CAD build for the part. Positions are in the model's coordinates, mm. Face numbers are marked on the shaded views. A direction names the side the tool comes from. Round coordinates to 2 decimals unless told otherwise and drop trailing zeros. Write each loop counter-clockwise with the first axis right and the second up, starting at its lowest first coordinate (ties: lowest second). Pieces come first, ordered by that corner, then holes. Notation, with made-up numbers: (-18, 83.5) - (26, 83.5) arc R25 cw to (26, 106.5) - close; hole circle Ø3 at (34, -25). An arc over 180 degrees is marked (long way). Answer in a Markdown table with one row per item.
```python
from build123d import *

# Parameters (mm, degrees)
SKETCH1_W               = 402.68
SKETCH1_H               = 30
BOSS_EXTRUDE1_DEPTH     = 2.03
SKETCH2_W               = 402.68
SKETCH2_H               = 30
BOSS_EXTRUDE2_DEPTH     = 2.03
CONVERT_SOLID1_START    = -201.34
CONVERT_SOLID1_DEPTH    = 402.68
CONVERT_SOLID1_2_DEPTH  = 402.68
CUT_EXTRUDE1_START      = -201.34
CUT_EXTRUDE1_DEPTH      = 75
CUT_EXTRUDE1_START_2    = 126.34
CUT_EXTRUDE1_2_DEPTH    = 75
CUT_EXTRUDE2_DEPTH      = 239.296116766
CUT_EXTRUDE2_DEPTH_BACK = 239.296116766
SKETCH8_R               = 3.1
CUT_EXTRUDE3_DEPTH      = 239.27017557
CUT_EXTRUDE3_DEPTH_BACK = 239.27017557
SKETCH10_R              = 3.1


# Read off the part's stored shape, not the designer's step: Convert-Solid1, Cut-Extrude1
with BuildPart() as part:
    # Sketch1 → Boss-Extrude1 (new body)
    with BuildSketch(Plane(origin=(0, 0, 0), x_dir=(1, 0, 0), z_dir=(0, 1, 0))):
        Rectangle(SKETCH1_W, SKETCH1_H)
    extrude(amount=BOSS_EXTRUDE1_DEPTH)


with BuildPart() as body_2:
    # Sketch2 → Boss-Extrude2 (new body)
    with BuildSketch(Plane(origin=(0, 0, 0), x_dir=(1, 0, 0), z_dir=(0, 1, 0))):
        with Locations((0, 112.4)):
            Rectangle(SKETCH2_W, SKETCH2_H)
    extrude(amount=-BOSS_EXTRUDE2_DEPTH)


    add(part.part)  # loft1 joins it to this body
    # loft from a face of the part (loft1)
    loft([body_2.faces().sort_by_distance((0, -1.015, -97.4))[0], body_2.faces().sort_by_distance((0, 1.015, -15))[0]])

    # Convert-Solid1 outline → Convert-Solid1 (cut)
    with BuildSketch(Plane.YZ.offset(CONVERT_SOLID1_START)):
        with BuildLine():
            ThreePointArc((2.03, -14.851837405), (2.029087712, -14.999988764), (2.026350985, -15.148117654))
            Line((2.026350985, -15.148117654), (2.03, -15))
            Line((2.03, -15), (2.03, -14.851837405))
        make_face()
        with BuildLine():
            ThreePointArc((-2.03, -97.523160927), (-2.029683266, -97.435865309), (-2.02873308, -97.348574287))
            Line((-2.02873308, -97.348574287), (-2.03, -97.4))
            Line((-2.03, -97.4), (-2.03, -97.523160927))
        make_face()
    extrude(amount=CONVERT_SOLID1_DEPTH, mode=Mode.SUBTRACT)

    # Convert-Solid1 2 outline → Convert-Solid1 2 (add)
    with BuildSketch(Plane.YZ.offset(CONVERT_SOLID1_START)):
        with BuildLine():
            Line((0, -97.4), (0, -97.523160927))
            ThreePointArc((0, -97.523160927), (0.000758344, -97.40000934), (0.003033263, -97.276876431))
            Line((0.003033263, -97.276876431), (0, -97.4))
        make_face()
        with BuildLine():
            ThreePointArc((0, -14.851837405), (-0.000758344, -14.974988992), (-0.003033263, -15.098121901))
            Line((-0.003033263, -15.098121901), (-2.026350985, -97.226880678))
            ThreePointArc((-2.026350985, -97.226880678), (-2.027695942, -97.28772447), (-2.02873308, -97.348574287))
            Line((-2.02873308, -97.348574287), (0, -15))
            Line((0, -15), (0, -14.851837405))
        make_face()
    extrude(amount=CONVERT_SOLID1_2_DEPTH)

    # Cut-Extrude1 outline → Cut-Extrude1 (cut)
    with BuildSketch(Plane.YZ.offset(CUT_EXTRUDE1_START)):
        with BuildLine():
            Line((-0.003033263, -15.098121901), (-1.508642262, -76.212497042))
            Line((-1.508642262, -76.212497042), (0.520741986, -76.262492795))
            Line((0.520741986, -76.262492795), (2.026350985, -15.148117654))
            ThreePointArc((2.026350985, -15.148117654), (2.029087712, -14.999988764), (2.03, -14.851837405))
            Line((2.03, -14.851837405), (2.03, -6.212497042))
            Line((2.03, -6.212497042), (0, -6.212497042))
            Line((0, -6.212497042), (0, -14.851837405))
            ThreePointArc((0, -14.851837405), (-0.000758344, -14.974988992), (-0.003033263, -15.098121901))
        make_face()
    extrude(amount=CUT_EXTRUDE1_DEPTH, mode=Mode.SUBTRACT)

    # Cut-Extrude1 2 outline → Cut-Extrude1 2 (cut)
    with BuildSketch(Plane.YZ.offset(CUT_EXTRUDE1_START_2)):
        with BuildLine():
            Line((-0.003033263, -15.098121901), (-1.508642262, -76.212497042))
            Line((-1.508642262, -76.212497042), (0.520741986, -76.262492795))
            Line((0.520741986, -76.262492795), (2.026350985, -15.148117654))
            ThreePointArc((2.026350985, -15.148117654), (2.029087712, -14.999988764), (2.03, -14.851837405))
            Line((2.03, -14.851837405), (2.03, -6.212497042))
            Line((2.03, -6.212497042), (0, -6.212497042))
            Line((0, -6.212497042), (0, -14.851837405))
            ThreePointArc((0, -14.851837405), (-0.000758344, -14.974988992), (-0.003033263, -15.098121901))
        make_face()
    extrude(amount=CUT_EXTRUDE1_2_DEPTH, mode=Mode.SUBTRACT)

    # Sketch8 → Cut-Extrude2 (cut, two sides: drawn at the far end of the back side and taken through both)
    with BuildSketch(Plane.XZ.offset(2.03).offset(-CUT_EXTRUDE2_DEPTH_BACK)):
        with Locations(Location((95.117, -114.9, 0), (0, 0, 270))):
            Circle(SKETCH8_R)
        with Locations(Location((-95.117, -114.9, 0), (0, 0, 270))):
            Circle(SKETCH8_R)
    extrude(amount=CUT_EXTRUDE2_DEPTH + CUT_EXTRUDE2_DEPTH_BACK, mode=Mode.SUBTRACT)

    # Sketch10 → Cut-Extrude3 (cut, two sides: drawn at the far end of the back side and taken through both)
    with BuildSketch(Plane.XZ.offset(-CUT_EXTRUDE3_DEPTH_BACK)):
        with Locations(Location((95.116996944, 2.5, 0), (0, 0, 270))):
            Circle(SKETCH10_R)
        with Locations(Location((-95.117, 2.5, 0), (0, 0, 270))):
            Circle(SKETCH10_R)
    extrude(amount=CUT_EXTRUDE3_DEPTH + CUT_EXTRUDE3_DEPTH_BACK, mode=Mode.SUBTRACT)


solid = body_2.part
```
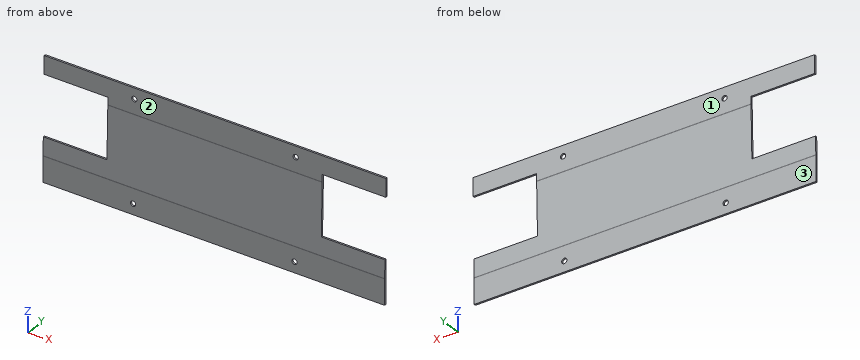
Q1. Saw through at D-D on z = -60. List the corners of the cut face in (x, y), then the cut area to 3 significant figures.
Computed:
| item | result |
|---|---|
| outline | (-126.34, -1.11) - (126.34, -1.11) - (126.34, 0.92) - (-126.34, 0.92) - close |
| area | 513 mm2 |
Q2. Saw through at C-C on x = 40. List the corners of the cut face in (y, z).
Computed:
| item | result |
|---|---|
| outline | (-2.03, -127.4) - (0, -127.4) - (0, -97.52) arc R10 cw to (0, -97.28) - (2.03, -15.15) arc R12.03 ccw to (2.03, -14.85) - (2.03, 15) - (0, 15) - (0, -14.85) arc R10 cw to (0, -15.1) - (-2.03, -97.23) arc R12.03 ccw to (-2.03, -97.35) arc R12.03 ccw to (-2.03, -97.52) - close |
Q3. Drill centre lines: line 1 (X direction, y = -0.55, z = -114.9); line 2 (Y direction, x = -47, z = -7.5); line 3 (Z direction, x = -144, y = -1). Where is each one in solid material? Low to high.
Computed:
| item | result |
|---|---|
| line 1 | x = -201.34 to -98.22, -92.02 to 92.02, 98.22 to 201.34 |
| line 2 | y = 0 to 2.03 |
| line 3 | z = -127.4 to -76.23 |
Q4. Saw through at B-B on y = 1.35. List the corners of the cut face in (x, z).
Computed:
| item | result |
|---|---|
| outline | (-201.34, -6.21) - (-126.34, -6.21) - (-126.34, -42.6) - (126.34, -42.6) - (126.34, -6.21) - (201.34, -6.21) - (201.34, 15) - (-201.34, 15) - close; hole circle Ø6.2 at (-95.12, 2.5); hole circle Ø6.2 at (95.12, 2.5) |
Q5. Flat gauge pins, fed straight in: pin 1 (8 mm diameter, centred on x = -95.117, z = -114.9, fed in from +Y); pin 2 (0.6 mm diameter, centred on x = -177.5, y = 1, fed in from -Z); pin 3 (6 mm diameter, centred on x = -3.5, z = -64.5, fed in from +Y). Where does each tip first touch, or does it go through?
Computed:
| item | result |
|---|---|
| pin 1 | stops at y = 0 |
| pin 2 | stops at z = -6.21 |
| pin 3 | stops at y = 0.88 |
Q6. Saw through at A-A on x = -139. List the corners of the cut face in (y, z).
Computed:
| item | result |
|---|---|
| outline | (-2.03, -127.4) - (0, -127.4) - (0, -97.52) arc R10 cw to (0, -97.28) - (0.52, -76.26) - (-1.51, -76.21) - (-2.03, -97.23) arc R12.03 ccw to (-2.03, -97.35) arc R12.03 ccw to (-2.03, -97.52) - close; (0, -6.21) - (2.03, -6.21) - (2.03, 15) - (0, 15) - close |
Q7. 3-axis set-ups, long thin cutter, end or side, ignore diameter. For the marked faces 1, 2 and 3: which of +Z, -Z, +X, -X, +Y, -Y reach the whole face in a straight line?
Computed:
| item | result |
|---|---|
| face 1 | +Z, -Z, +X, -X, +Y |
| face 2 | +Z, +X, -X, -Y |
| face 3 | -Z, +X, -X, +Y |
